```python
from build123d import *

# Parameters (mm, degrees)
F0_W     = 15
F0_H     = 60
F1_DEPTH = 7
F0_R     = 2.05
F2_DEPTH = 3.7


with BuildPart() as f1:
    # F0 (on Top) → F1 (new body)
    with BuildSketch(Plane.XY):
        Rectangle(F0_W, F0_H)
        Polygon((-2.049593, -20.95), (2.049593, -20.95), (4.099187, -24.5), (2.049593, -28.05), (-2.049593, -28.05), (-4.099187, -24.5), align=None, mode=Mode.SUBTRACT)
        Polygon((4.099187, 24.5), (2.049593, 20.95), (-2.049593, 20.95), (-4.099187, 24.5), (-2.049593, 28.05), (2.049593, 28.05), align=None, mode=Mode.SUBTRACT)
    extrude(amount=F1_DEPTH)

    # F0 (on Top) → F2 (join)
    with BuildSketch(Plane.XY):
        Polygon((4.099187, -24.5), (2.049593, -20.95), (-2.049593, -20.95), (-4.099187, -24.5), (-2.049593, -28.05), (2.049593, -28.05), align=None)
        with Locations((0, -24.5)):
            Circle(F0_R, mode=Mode.SUBTRACT)
        Polygon((-2.049593, 20.95), (2.049593, 20.95), (4.099187, 24.5), (2.049593, 28.05), (-2.049593, 28.05), (-4.099187, 24.5), align=None)
        with Locations((0, 24.5)):
            Circle(F0_R, mode=Mode.SUBTRACT)
    extrude(amount=F2_DEPTH)


solid = f1.part
```
Design review of the part built by this model. Coordinates are the model's own, in mm. A direction names the side the tool comes from. Give positions to 0.01 mm unless a question says otherwise; leave off trailing zeros. Loops run counter-clockwise (first coordinate to the right, second up) from the corner with the lowest first, then second, coordinate; pieces in that order, holes last. Notation, with made-up numbers: (-1.5, 56.25) -> (43.5, 56.25) arc R23 ccw to (43.5, 81.25) -> close; hole circle Ø7 at (-1.75, 30.25). An arc over 180 degrees is marked (long way). Write each question's results on one line, items separated by ' | '.
Q1. The part is to be moulded in two halves that separate along Y. For faces 1 (the face through (0, -30, 3)), 2 (the face through (0, 0, 0)), 3 (the face through (3.06, 26.3, 5.33)), 4 (the face through (0, 20.95, 5)), say which applies: +Y half, -Y half, draft (parallel to the pull), parting line (faces both ways), or undercut.
Reply:
face 1: -Y half | face 2: draft | face 3: undercut | face 4: undercut
Q2. Machinability: for faces 5 (the face through (3.06, -22.7, 5.33)), 6 (the face through (7.5, 0, 3)), which of the approach directions +Z, -Z, +X, -X, +Y, -Y give a long, thin tool a straight path to every point of the face, cutting with its end or side? Answer none if there is none.
Reply:
face 5: +Z | face 6: +Z, -Z, +X, +Y, -Y
Q3. Take a section at D-D, the plane z = 2.5. Write out the cut boundary in (x, y), plus the area to 3 significant figures.
Reply:
outline: (-7.5, -30) -> (7.5, -30) -> (7.5, 30) -> (-7.5, 30) -> close; hole circle Ø4.1 at (0, -24.5); hole circle Ø4.1 at (0, 24.5) | area: 874 mm²
Q4. Take a section at C-C, the plane x = 3. Write out the cut boundary in (y, z), plus the area to 3 significant figures.
Reply:
outline: (-30, 0) -> (30, 0) -> (30, 7) -> (26.4, 7) -> (26.4, 3.7) -> (22.6, 3.7) -> (22.6, 7) -> (-22.6, 7) -> (-22.6, 3.7) -> (-26.4, 3.7) -> (-26.4, 7) -> (-30, 7) -> close | area: 395 mm²
Q5. Wall thickness on L1, parallel to Y at x = 0, z = 1.8; L2, parallel to Y at x = 2, z = 6.5; L3, parallel to Z at x = 2.25, y = 23.5: over which ranges is each line inside the solid? List them lowest first.
Reply:
L1: y = -30 to -26.55, -22.45 to 22.45, 26.55 to 30 | L2: y = -30 to -28.05, -20.95 to 20.95, 28.05 to 30 | L3: z = 0 to 3.7
Q6. Take a section at B-B, the plane z = 6.5. Write out the cut boundary in (x, y).
Reply:
outline: (-7.5, -30) -> (7.5, -30) -> (7.5, 30) -> (-7.5, 30) -> close; hole (-4.1, -24.5) -> (-2.05, -28.05) -> (2.05, -28.05) -> (4.1, -24.5) -> (2.05, -20.95) -> (-2.05, -20.95) -> close; hole (-4.1, 24.5) -> (-2.05, 20.95) -> (2.05, 20.95) -> (4.1, 24.5) -> (2.05, 28.05) -> (-2.05, 28.05) -> close
Q7. For pin 1 Ø2 at (x, y) = (-1, 13.5) entering from -Z; pin 2 Ø2 at (x, y) = (-1, -25) entering from +Z, all flat-tipped, find the tip position at first contact; note any pin that passes through.
Reply:
pin 1: stops at z = 0 | pin 2: stops at z = 3.7
Q8. Take a section at A-A, the plane x = 0. Write out the cut boundary in (y, z), plus the area to 3 significant figures.
Reply:
outline: (-30, 0) -> (-26.55, 0) -> (-26.55, 3.7) -> (-28.05, 3.7) -> (-28.05, 7) -> (-30, 7) -> close; (-22.45, 0) -> (22.45, 0) -> (22.45, 3.7) -> (20.95, 3.7) -> (20.95, 7) -> (-20.95, 7) -> (-20.95, 3.7) -> (-22.45, 3.7) -> close; (26.55, 0) -> (30, 0) -> (30, 7) -> (28.05, 7) -> (28.05, 3.7) -> (26.55, 3.7) -> close | area: 343 mm²
